Geometry check sheet. Reference: the model listing, model coordinates, mm. Face numbers are marked on the shaded views. A direction names the side the tool comes from. Round coordinates to 2 decimals unless told otherwise and drop trailing zeros. Write each loop counter-clockwise with the first axis right and the second up, starting at its lowest first coordinate (ties: lowest second). Pieces come first, ordered by that corner, then holes.
Item 1: Access from +Z, -Z, +X, -X, +Y, -Y to the whole of each face (thin tool, end or side, straight path). Record for the marked faces 1 and 2.
Item 2: Scan lines: probe 1 along Y at (x, z) = (1, 2.75) (3 decimals); probe 2 along X at (y, z) = (2, -0.75); probe 3 along X at (y, z) = (3.5, 0.25). Record each from-to range of solid material in increasing order.
Item 3: Depth check by flat-ended pin: P1, Ø2, axis at x = 2.5, y = -1.5, coming from the -Z side; P2, Ø3, axis at y = 3.5, z = 2, coming from the -X side. Enter the tip coordinate at first touch or a pass-through.
Item 4: Cross-section at C-C (y = 3.5). Enter the section's corners in (x, z), then the cut area to 3 significant figures.
Item 5: Cross-section at A-A (z = 0). Enter the section's corners in (x, y) (3 decimals), then the cut area to 3 significant figures.
Item 6: Cross-section at B-B (x = 0). Enter the section's corners in (y, z) (3 decimals).
Item 7: Cross-section at D-D (y = -1.5). Enter the section's corners in (x, z).
Autodesk Inventor part; units mm, degrees
ref_plane "YZ Plane" through (0, 0, 0) normal (1, 0, 0) x (0, 1, 0)
ref_plane "XZ Plane" through (0, 0, 0) normal (0, 1, 0) x (-1, 0, 0)
ref_plane "XY Plane" through (0, 0, 0) normal (0, 0, 1) x (1, 0, 0)
sketch "Sketch1" plane through (0, 0, 0) normal (0, 1, 0) x (-1, 0, 0)
  circle A0 centre (0, 0) radius 3.6513
  circle A1 centre (0, 0) radius 2.6987
  dimension "d0" = 7.3025
  dimension "d1" = 5.3975
extrude "Extrusion1" add sketch "Sketch1" along normal blind 6.35 contours A1
extrude "Extrusion2" add sketch "Sketch1" along normal blind 3.175
extrude "Extrusion3" add sketch "Sketch1" against normal blind 4.445 contours A0 | A1
properties part number "Track v3 Button"
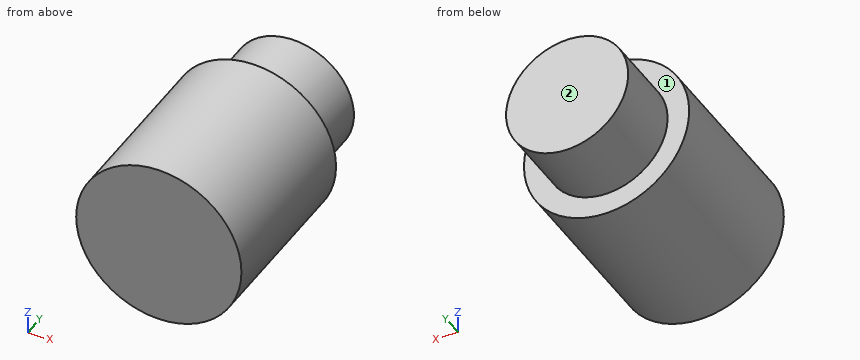
Resolved:
1. face 1: +Y
1. face 2: +Z, -Z, +X, -X, +Y
2. probe 1: y = -4.445 to 3.175
2. probe 2: x = -3.57 to 3.57
2. probe 3: x = -2.69 to 2.69
3. P1: stops at z = -3.33
3. P2: stops at x = -3.61
4. outline: circle Ø5.4 at (0, 0)
4. area: 22.9 mm2
5. outline: (-3.651, -4.445) - (3.651, -4.445) - (3.651, 3.175) - (2.699, 3.175) - (2.699, 6.35) - (-2.699, 6.35) - (-2.699, 3.175) - (-3.651, 3.175) - close
5. area: 72.8 mm2
6. outline: (-4.445, -3.651) - (3.175, -3.651) - (3.175, -2.699) - (6.35, -2.699) - (6.35, 2.699) - (3.175, 2.699) - (3.175, 3.651) - (-4.445, 3.651) - close
7. outline: circle Ø7.3 at (0, 0)
